from build123d import *

# Parameters (mm, degrees)
F1_DEPTH = 12.7
F2_W     = 76.2
F2_H     = 12.7
F3_DEPTH = 38.1
F4_W     = 76.2
F4_H     = 12.7
F5_DEPTH = 38.1
F6_W     = 76.2
F6_H     = 12.7
F7_DEPTH = 38.1
F8_W     = 76.2
F8_H     = 12.7
F9_DEPTH = 38.1


with BuildPart() as f1:
    # F0 (on Top) → F1 (new body)
    with BuildSketch(Plane.XY):
        Polygon((34.9385468854, 114.4016), (-52.5428857533, 114.4016), (-114.4016, 52.5428857533), (-114.4016, -34.9385468854), (-52.5428857533, -96.7972611321), (34.9385468854, -96.7972611321), (96.7972611321, -34.9385468854), (96.7972611321, 52.5428857533), align=None)
    extrude(amount=F1_DEPTH)

    # F2 (on face) → F3 (cut)
    with BuildSketch(Plane(origin=(65.8679040087, -65.8679040087, 0), x_dir=(0.7071067812, 0.7071067812, 0), z_dir=(0.7071067812, -0.7071067812, 0))):
        with Locations((0, 6.35)):
            Rectangle(F2_W, F2_H)
    extrude(amount=-F3_DEPTH, mode=Mode.SUBTRACT)

    # F4 (on face) → F5 (cut)
    with BuildSketch(Plane(origin=(-74.6700734427, -74.6700734427, 0), x_dir=(0.7071067812, -0.7071067812, 0), z_dir=(-0.7071067812, -0.7071067812, 0))):
        with Locations((-12.4481473918, 6.35)):
            Rectangle(F4_W, F4_H)
    extrude(amount=-F5_DEPTH, mode=Mode.SUBTRACT)

    # F6 (on face) → F7 (cut)
    with BuildSketch(Plane(origin=(-83.4722428766, 83.4722428766, 0), x_dir=(-0.7071067812, -0.7071067812, 0), z_dir=(-0.7071067812, 0.7071067812, 0))):
        with Locations((0, 6.35)):
            Rectangle(F6_W, F6_H)
    extrude(amount=-F7_DEPTH, mode=Mode.SUBTRACT)

    # F8 (on face) → F9 (cut)
    with BuildSketch(Plane(origin=(74.6700734427, 74.6700734427, 0), x_dir=(-0.7071067812, 0.7071067812, 0), z_dir=(0.7071067812, 0.7071067812, 0))):
        with Locations((12.4481473918, 6.35)):
            Rectangle(F8_W, F8_H)
    extrude(amount=-F9_DEPTH, mode=Mode.SUBTRACT)


solid = f1.part
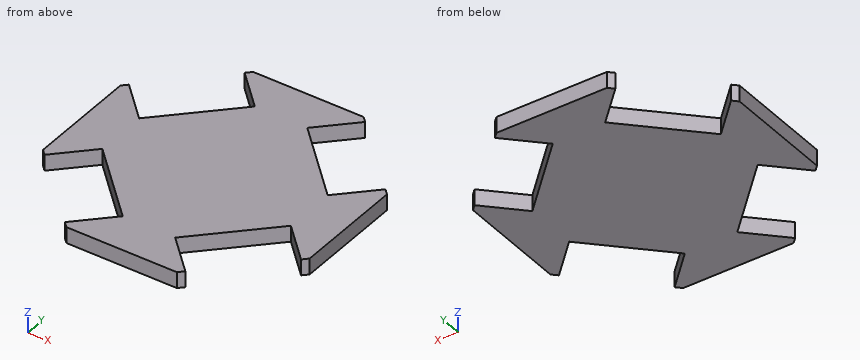
Could you check a few things on this model? Use its own coordinates, in mm. Give positions to 0.01 mm unless a question says otherwise; leave off trailing zeros. Write each loop counter-clockwise with the first axis right and the second up, starting at its lowest first coordinate (ties: lowest second). Pieces come first, ordered by that corner, then holes. Notation, with made-up numbers: (-32.5, -24) -> (-28.5, -24) arc R12 ccw to (-28.5, -11) -> close; hole circle Ø2 at (64.25, 38). An arc over 180 degrees is marked (long way). Write each question's results on one line, items separated by ' | '. Start each with the question number.
Q1. I need wall thicknesses on probe 1 along X at (y, z) = (-29, 12.25); probe 2 along X at (y, z) = (-22, 9); probe 3 along Y at (x, z) = (23.5, 2). Which ranges of each line are inside material? Lowest first, please.
Q2. I'm going to push flat-ended pins straight in: pin 1 Ø1 at (x, z) = (53.5, 1.5) entering from +Y; pin 2 Ø4 at (y, z) = (78, 4.5) entering from -X. Where does each tip first touch, or does it pass through?
Q3. Suppose I cut it at B-B, the plane z = 7.5. List the corners of the cut face in (x, y) for me, and give its area (3 significant figures).
Q4. Suppose I cut it at D-D, the plane y = 60.5. List the corners of the cut face in (x, z) for me.
Q5. Suppose I cut it at A-A, the plane x = -42. List the corners of the cut face in (y, z) for me, and give its area (3 significant figures).
Q6. Suppose I cut it at C-C, the plane x = -87.5. List the corners of the cut face in (y, z) for me, and give its area (3 significant figures).
Outcome:
1) probe 1: -114.4 to -100.49, -66.46 to 48.85, 82.88 to 96.8 | probe 2: -114.4 to -93.49, -73.46 to 55.85, 75.88 to 96.8 | probe 3: -96.8 to -77.38, -54.35 to 71.96, 94.99 to 114.4
2) pin 1: y = 42.46 | pin 2: x = -37.06
3) outline: (-114.4, -34.94) -> (-110.41, -38.93) -> (-83.47, -11.99) -> (-29.59, -65.87) -> (-56.53, -92.81) -> (-52.54, -96.8) -> (34.94, -96.8) -> (38.93, -92.81) -> (11.99, -65.87) -> (65.87, -11.99) -> (92.81, -38.93) -> (96.8, -34.94) -> (96.8, 52.54) -> (92.81, 56.53) -> (65.87, 29.59) -> (11.99, 83.47) -> (38.93, 110.41) -> (34.94, 114.4) -> (-52.54, 114.4) -> (-56.53, 110.41) -> (-29.59, 83.47) -> (-83.47, 29.59) -> (-110.41, 56.53) -> (-114.4, 52.54) -> close | area: 25,300 mm2
4) outline: (-52.56, 0) -> (34.96, 0) -> (34.96, 12.7) -> (-52.56, 12.7) -> close
5) outline: (-96.8, 0) -> (-78.28, 0) -> (-78.28, 12.7) -> (-96.8, 12.7) -> close; (-53.46, 0) -> (71.06, 0) -> (71.06, 12.7) -> (-53.46, 12.7) -> close; (95.88, 0) -> (114.4, 0) -> (114.4, 12.7) -> (95.88, 12.7) -> close | area: 2,050 mm2
6) outline: (-16.01, 0) -> (33.62, 0) -> (33.62, 12.7) -> (-16.01, 12.7) -> close | area: 630 mm2
